Geometry: see drawing. Coordinates: mm, zero at the bounding-box minimum. A direction names the side the tool comes from. Round coordinates to 2 decimals unless told otherwise and drop trailing zeros. Loops run counter-clockwise (first coordinate to the right, second up) from the corner with the lowest first, then second, coordinate; pieces in that order, holes last. Notation, with made-up numbers: (73, 53.5) - (132, 53.5) arc R12 cw to (132, 63.5) - close; hole circle Ø4 at (-26.5, -13.75). An arc over 180 degrees is marked (long way). Use CSV: the item, a comma, the result in double quotes. Start each with the question number.
1. Cut plane D-D (z = 11). Return loops of the section in (x, y) (1 decimal), and give its area (3 significant figures).
2. Pull-direction query (Z, two-part tool) for the marked faces 4, 5 and 6; classes: +Z half, -Z half, draft (parallel to the pull), parting line (faces both ways), or undercut.
3. Cut plane A-A (z = 29). Return loops of the section in (x, y) (1 decimal), and give its area (3 significant figures).
4. Cut plane C-C (y = 35). Return loops of the section in (x, z) (1 decimal).
5. Pin query (flat end, axial travel): P1, Ø10, axis at x = 4, y = 41.5, coming from the +Z side; P2, Ø2, axis at x = 50, z = 30, coming from the -Y side; P3, Ø8, axis at y = 36, z = 30.5, coming from the -X side; P4, Ø5, axis at x = 28.5, y = 48, coming from the +Z side. Return the tip coordinate at first contact, or that it passes through.
6. Material intervals for probe 1 along X at (y, z) = (15.75, 29) (1 decimal); probe 2 along Z at (x, y) = (28, 43.5); probe 3 along X at (y, z) = (14.75, 29) (1 decimal), sorted ascending. Write a range as from..to.
7. Cut plane B-B (x = 51). Return loops of the section in (y, z).
8. Access query for the marked faces 1, 2 and 3. Directions: +Z, -Z, +X, -X, +Y, -Y. A direction counts if a zero-diameter tool reaches every point of the face in a straight line with its end or side. Return the directions, or none.
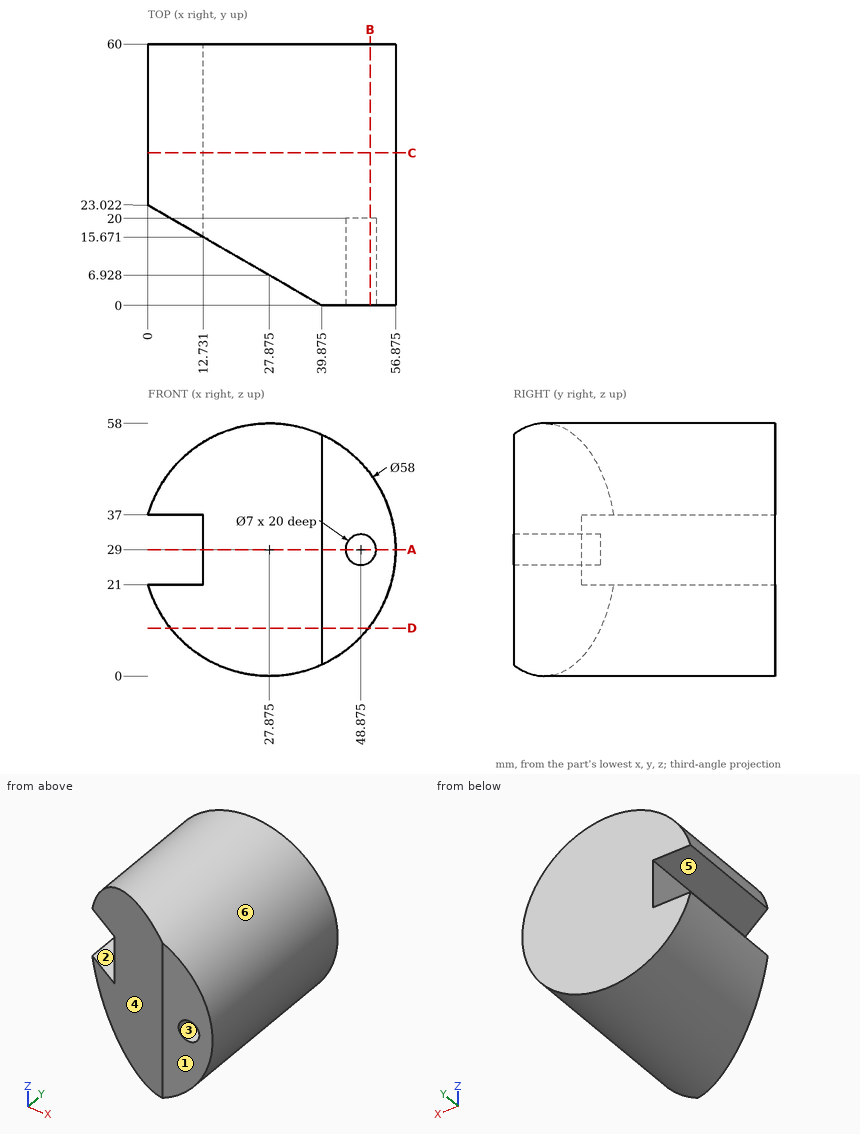
Established:
1,outline,"(5.1, 20.1) - (39.9, 0) - (50.6, 0) - (50.6, 60) - (5.1, 60) - close"
1,area,"2,380 mm2"
2,face 4,"draft"
2,face 5,"undercut"
2,face 6,"parting line"
3,outline,"(12.7, 15.7) - (39.9, 0) - (45.4, 0) - (45.4, 20) - (52.4, 20) - (52.4, 0) - (56.9, 0) - (56.9, 60) - (12.7, 60) - close"
3,area,"2,300 mm2"
4,outline,"(0, 21) arc R29 ccw (long way) to (0, 37) - (12.7, 37) - (12.7, 21) - close"
5,P1,"stops at z = 51.02"
5,P2,"stops at y = 20"
5,P3,"stops at x = 12.73"
5,P4,"stops at z = 58"
6,probe 1,"x = 12.7..45.4, 52.4..56.9"
6,probe 2,"z = 0..58"
6,probe 3,"x = 14.3..45.4, 52.4..56.9"
7,outline,"(0, 11.5) - (60, 11.5) - (60, 46.5) - (0, 46.5) - (0, 31.78) - (20, 31.78) - (20, 26.22) - (0, 26.22) - close"
8,face 1,"+Z, -Z, +X, -X, -Y"
8,face 2,"-X, +Y, -Y"
8,face 3,"-Y"
